Study the drawing (mm; zero at the part's minimum x, y, z) and answer. Coordinates: 2 decimals unless noted, no trailing zeros. Order: outer loops, then holes, each group sorted by start corner. A loop starts at its lowest first (then second) coordinate and runs counter-clockwise, first axis right, second up. Notation, with made-up numbers: M -30.5,4 L 27.5,4 A18 ccw 27.5,18 Z; hole C -22,26 d8. An arc over 180 degrees is marked long. Use a Markdown table: item, result. Add a question column.
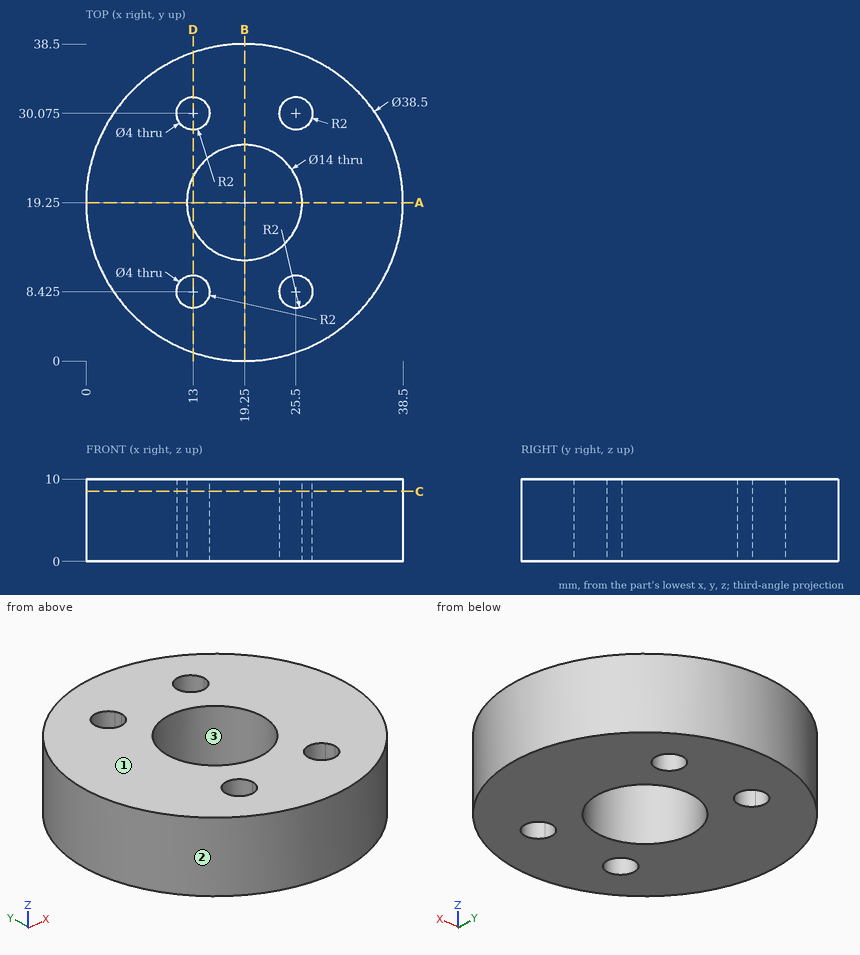
(1) The mould has two halves that part along Y. Classify the marked faces 1, 2 and 3: pulls with the +Y half, pulls with the -Y half, needs draft (parallel to the pull), parting line crosses it, or undercut.
(2) Given P1, Ø8.5, axis at x = 19.25, y = 19.25, coming from the +Z side (3 decimals); P2, Ø6, axis at y = 25, z = 8.5, coming from the +X side; P3, Ø5, axis at y = 14.5, z = 8.5, coming from the -X side; P4, Ø5, axis at y = 5.5, z = 8, coming from the +X side, each flat-ended and moving along its own axis, determine where each tip first touches the part or whether it passes through.
(3) Straight lines are drawn through the part: line 1 (Y direction, x = 19.5, z = 4) (1 decimal); line 2 (Y direction, x = 14.5, z = 6.75) (1 decimal). For each, find the intervals that lie inside material, in ascending order.
(4) A cutting plane is placed at A-A on y = 19.25. Write down the section's boundary in (x, z), plus the area to 3 significant figures.
(5) A cutting plane is placed at C-C on z = 8.5. Count the separate pieces of the cut face and the enclosed holes in it, plus the area to 3 significant figures.
(6) A cutting plane is placed at D-D on x = 13. Write down the section's boundary in (y, z) (1 decimal), plus the area to 3 significant figures.
From the geometry:
| question | item | result |
|---|---|---|
| 1 | face 1 | needs draft |
| 1 | face 2 | parting line crosses it |
| 1 | face 3 | undercut |
| 2 | P1 | passes through |
| 2 | P2 | stops at x = 38.3 |
| 2 | P3 | stops at x = 0.13 |
| 2 | P4 | stops at x = 34.87 |
| 3 | line 1 | y = 0 to 12.3, 26.2 to 38.5 |
| 3 | line 2 | y = 0.6 to 7.1, 9.7 to 14.1, 24.4 to 28.8, 31.4 to 37.9 |
| 4 | outline | M 0,0 L 12.25,0 L 12.25,10 L 0,10 Z; M 26.25,0 L 38.5,0 L 38.5,10 L 26.25,10 Z |
| 4 | area | 245 mm2 |
| 5 | separate pieces | 1 |
| 5 | enclosed holes | 5 |
| 5 | area | 960 mm2 |
| 6 | outline | M 1,0 L 6.4,0 L 6.4,10 L 1,10 Z; M 10.4,0 L 16.1,0 L 16.1,10 L 10.4,10 Z; M 22.4,0 L 28.1,0 L 28.1,10 L 22.4,10 Z; M 32.1,0 L 37.5,0 L 37.5,10 L 32.1,10 Z |
| 6 | area | 221 mm2 |
